```python
from build123d import *

# Parameters (mm, degrees)
F1_DEPTH = 20.32
F2_W     = 3.1245226281
F2_H     = 8.89
F6_D     = 11.1125


with BuildPart() as f1:
    # F0 (on Top) → F1 (new body)
    with BuildSketch(Plane.XY):
        Polygon((-9.525, 5.499261314), (-9.525, -5.499261314), (0, -10.9985226281), (9.525, -5.499261314), (9.525, 5.499261314), (0, 10.9985226281), align=None)
    extrude(amount=-F1_DEPTH)

    # F2 (on Right) → F4 (revolve, cut)
    with BuildSketch(Plane.YZ):
        with Locations((-9.436261314, -15.875)):
            Rectangle(F2_W, F2_H)
    revolve(axis=Axis((0, 0, -8.0978884362), (0, 0, -1)), mode=Mode.SUBTRACT)

    # F6 (through all)
    with Locations(Plane.XY):
        with Locations((0, 0)):
            Hole(F6_D / 2)


solid = f1.part
```
Geometry check sheet. Reference: the model listing, model coordinates, mm. A direction names the side the tool comes from. Round coordinates to 2 decimals unless told otherwise and drop trailing zeros. Order: outer loops, then holes, each group sorted by start corner. A loop starts at its lowest first (then second) coordinate and runs counter-clockwise, first axis right, second up. Notation, with made-up numbers: M 65.25,37.5 L 103.25,37.5 A29 ccw 103.25,73.5 Z; hole C -35,-2 d8. An arc over 180 degrees is marked long. Answer as CSV lines item,"result".
1) Tool access check on faces 4 (the face through (8, -2, -11.43)), 5 (the face through (-4.696, 8.287, -5.635)). Record the directions out of +Z, -Z, +X, -X, +Y, -Y that give a thin tool (end or side, any length) a straight path to the whole face; none if there is none.
Entries:
face 4,"-Z"
face 5,"+Z, -Z, -X, +Y"
2) Gauge pin test, flat ends, axial feed: pin 1 Ø5 at (y, z) = (5, -16.5) entering from -X; pin 2 Ø10 at (x, y) = (-2.5, -4) entering from -Z; pin 3 Ø1.5 at (y, z) = (7.5, -9) entering from +X; pin 4 Ø8 at (x, z) = (0.5, -4.5) entering from -Y. Record the tip position at first contact, or that the pin passes through.
Entries:
pin 1,"x = -7.47"
pin 2,"z = -20.32"
pin 3,"x = 7.36"
pin 4,"y = -11"
3) Thickness scan on probe 1 along Y at (x, z) = (0, -12.5); probe 2 along X at (y, z) = (2.25, -6) (3 decimals); probe 3 along Y at (x, z) = (-3, -18.5). Record the ranges inside material, lowest first. Write a range as [from, to].
Entries:
probe 1,"[-7.87, -5.56], [5.56, 7.87]"
probe 2,"[-9.525, -5.08], [5.08, 9.525]"
probe 3,"[-7.28, -4.68], [4.68, 7.28]"
4) Sectioned sample at A-A on y = 0. Record the cut outline in (x, z) (3 decimals), and give its area (3 significant figures).
Entries:
outline,"M -9.525,-11.43 L -7.874,-11.43 L -7.874,-20.32 L -5.556,-20.32 L -5.556,0 L -9.525,0 Z; M 5.556,-20.32 L 7.874,-20.32 L 7.874,-11.43 L 9.525,-11.43 L 9.525,0 L 5.556,0 Z"
area,"132 mm2"
5) Sectioned sample at C-C on y = -2.75. Record the cut outline in (x, z) (3 decimals).
Entries:
outline,"M -9.525,-11.43 L -7.378,-11.43 L -7.378,-20.32 L -4.828,-20.32 L -4.828,0 L -9.525,0 Z; M 4.828,-20.32 L 7.378,-20.32 L 7.378,-11.43 L 9.525,-11.43 L 9.525,0 L 4.828,0 Z"
6) Sectioned sample at B-B on z = -9.75. Record the cut outline in (x, y) (1 decimal).
Entries:
outline,"M -9.5,-5.5 L 0,-11 L 9.5,-5.5 L 9.5,5.5 L 0,11 L -9.5,5.5 Z; hole C 0,0 d11.1"
7) Mould release check, pull along Y, two halves, no side actions. Record for faces 1 (the face through (4.83, 8.21, -5.63)), 2 (the face through (-5.3, 1.67, -10.3)), 3 (the face through (4, -5, 0)): +Y half, -Y half, draft (parallel to the pull), parting line (faces both ways), or undercut.
Entries:
face 1,"+Y half"
face 2,"undercut"
face 3,"draft"
8) Sectioned sample at D-D on z = -12. Record the cut outline in (x, y).
Entries:
outline,"C 0,0 d15.75; hole C 0,0 d11.11"
